Can you work these out from the model? Positions are in its coordinate system, mm. A direction names the side the tool comes from. Round coordinates to 2 decimals unless told otherwise and drop trailing zeros. Write each loop counter-clockwise with the first axis right and the second up, starting at its lowest first coordinate (ties: lowest second). Pieces come first, ordered by that corner, then holes. Notation, with made-up numbers: (21.25, -38.5) -> (33.25, -38.5) arc R22 cw to (33.25, -30.5) -> close; hole circle Ø1 at (-33, -12.5). An arc over 180 degrees is marked (long way). Use CSV: the item, a comma, the result in double quotes.
```python
from build123d import *

# Parameters (mm, degrees)
F0_W     = 88.9625
F0_H     = 17.849998
F0_R     = 3.20625
F0_W_2   = 63.4375
F0_H_2   = 13.087498
F1_DEPTH = 7.9375
F3_R     = 4
F4_DEPTH = 6.35
F5_R     = 1.35255
F6_DEPTH = 4.7625
F7_R     = 1.5875
F8_R     = 6.381242


with BuildPart() as f1:
    # F0 (on Top) → F1 (new body)
    with BuildSketch(Plane.XY):
        Rectangle(F0_W, F0_H)
        with Locations((-38.1, 2.543749)):
            Circle(F0_R, mode=Mode.SUBTRACT)
        Rectangle(F0_W_2, F0_H_2, mode=Mode.SUBTRACT)
        with Locations((38.1, 2.543749)):
            Circle(F0_R, mode=Mode.SUBTRACT)
    extrude(amount=F1_DEPTH)

    # F3 (on face) → F4 (cut, through all)
    with BuildSketch(Plane.XY.offset(7.9375)):
        with Locations((-38.1, 2.543749)):
            Circle(F3_R)
        with Locations((38.1, 2.543749)):
            Circle(F3_R)
    extrude(amount=-F4_DEPTH, mode=Mode.SUBTRACT)

    # F5 (on face) → F6 (cut)
    with BuildSketch(Plane.XZ.offset(8.924999)):
        with Locations((-38.1, 3.96875)):
            Circle(F5_R)
        with Locations((38.1, 3.96875)):
            Circle(F5_R)
    extrude(amount=-F6_DEPTH, mode=Mode.SUBTRACT)

    # F7
    f7_edges = [f1.edges().sort_by_distance(p)[0] for p in [
        (31.71875, 6.543749, 3.96875),
        (31.71875, -6.543749, 3.96875),
        (-31.71875, -6.543749, 3.96875),
        (-31.71875, 6.543749, 3.96875),
    ]]
    fillet(f7_edges, radius=F7_R)

    # F8
    f8_edges = [f1.edges().sort_by_distance(p)[0] for p in [
        (44.48125, 8.924999, 3.96875),
        (-44.48125, 8.924999, 3.96875),
    ]]
    fillet(f8_edges, radius=F8_R)


solid = f1.part
```
Q1. Will these pins go through, and if not, where does the flat tip stop? P1, Ø2.5, axis at x = -38.5, y = 4, coming from the +Z side; P2, Ø2.5, axis at x = 36.5, y = 4, coming from the +Z side; P3, Ø1, axis at y = 7, z = 3, coming from the +X side.
Resolved:
P1,"passes through"
P2,"stops at z = 1.59"
P3,"stops at x = 43.11"
Q2. On a 3-axis mill with a long thin cutter (end or side, diameter ignored), from which of +Z, -Z, +X, -X, +Y, -Y can I reach the whole of each face in a straight line? I mean faces 5 (the face through (0, -7, 0)), 6 (the face through (35, 4, 1.588)), 7 (the face through (39.35, -6.58, 3.45)), 8 (the face through (0, 6.544, 4)). Say none if no direction works.
Resolved:
face 5,"-Z, +X, -X, +Y, -Y"
face 6,"+Z"
face 7,"-Y"
face 8,"+Z, -Z"
Q3. Suppose I cut it at B-B (z = 6.5). Write out the boundary of the cut face in (x, y) (1 decimal).
Resolved:
outline,"(-44.5, -8.9) -> (44.5, -8.9) -> (44.5, 2.5) arc R6.4 ccw to (38.1, 8.9) -> (-38.1, 8.9) arc R6.4 ccw to (-44.5, 2.5) -> close; hole circle Ø8 at (-38.1, 2.5); hole (-31.7, -5) arc R1.6 ccw to (-30.1, -6.5) -> (30.1, -6.5) arc R1.6 ccw to (31.7, -5) -> (31.7, 5) arc R1.6 ccw to (30.1, 6.5) -> (-30.1, 6.5) arc R1.6 ccw to (-31.7, 5) -> close; hole circle Ø8 at (38.1, 2.5)"
Q4. Suppose I cut it at D-D (x = -36). Write out the boundary of the cut face in (y, z) (1 decimal).
Resolved:
outline,"(-8.9, 0) -> (0.1, 0) -> (0.1, 1.6) -> (-0.9, 1.6) -> (-0.9, 7.9) -> (-8.9, 7.9) -> close; (5, 0) -> (8.9, 0) -> (8.9, 7.9) -> (5.9, 7.9) -> (5.9, 1.6) -> (5, 1.6) -> close"
Q5. Suppose I cut it at A-A (x = -2.5). Write out the boundary of the cut face in (y, z) (1 decimal), and give its area (3 significant figures).
Resolved:
outline,"(-8.9, 0) -> (-6.5, 0) -> (-6.5, 7.9) -> (-8.9, 7.9) -> close; (6.5, 0) -> (8.9, 0) -> (8.9, 7.9) -> (6.5, 7.9) -> close"
area,"37.8 mm^2"
Q6. Suppose I cut it at C-C (y = 0.25). Write out the boundary of the cut face in (x, z).
Resolved:
outline,"(-44.48, 0) -> (-40.34, 0) -> (-40.34, 1.59) -> (-41.38, 1.59) -> (-41.38, 7.94) -> (-44.48, 7.94) -> close; (-35.86, 0) -> (-31.72, 0) -> (-31.72, 7.94) -> (-34.82, 7.94) -> (-34.82, 1.59) -> (-35.86, 1.59) -> close; (31.72, 0) -> (35.86, 0) -> (35.86, 1.59) -> (34.82, 1.59) -> (34.82, 7.94) -> (31.72, 7.94) -> close; (40.34, 0) -> (44.48, 0) -> (44.48, 7.94) -> (41.38, 7.94) -> (41.38, 1.59) -> (40.34, 1.59) -> close"
Q7. Please list where these lines run through material, in increasing order: probe 1 along X at (y, z) = (-4, 4.75); probe 2 along Y at (x, z) = (3, 5) (3 decimals); probe 3 along X at (y, z) = (4.5, 5).
Resolved:
probe 1,"x = -44.48 to -31.72, 31.72 to 44.48"
probe 2,"y = -8.925 to -6.544, 6.544 to 8.925"
probe 3,"x = -44.17 to -41.59, -34.61 to -31.72, 31.72 to 34.61, 41.59 to 44.17"
Q8. If we mould it in two halves opening along Y, with no side actions, what happens to faces 1 (the face through (0, -7, 7.938)), 2 (the face through (-1, 8.925, 4)), 3 (the face through (-31.24, -6.09, 4.02)), 4 (the face through (-1, -8.925, 4))? For each: released by +Y, released by -Y, zero draft, split by the parting line, or undercut.
Resolved:
face 1,"zero draft"
face 2,"released by +Y"
face 3,"undercut"
face 4,"released by -Y"
